Geometry: see drawing. Coordinates: mm, zero at the bounding-box minimum. A direction names the side the tool comes from. Give positions to 0.01 mm unless a question says otherwise; leave off trailing zeros. Order: outer loops, then holes, each group sorted by start corner. A loop starts at its lowest first (then second) coordinate and runs counter-clockwise, first axis right, second up. Notation, with made-up numbers: M -13.5,5.5 L 40.5,5.5 A32 cw 40.5,38.5 Z; hole C 42.5,18.5 d2. An arc over 180 degrees is marked long. Answer as a JSON object with one key per item and string values. Group by question number.
1. Section query D-D (x = 22.5). Output: boundary loops of the cut face in (y, z).
2. Pin query (flat end, axial travel): P1, Ø1.8, axis at x = 23, y = 22.25, coming from the +Z side; P2, Ø0.6, axis at x = 7.5, z = 0.5, coming from the -Y side; P3, Ø1, axis at y = 6.5, z = 1.5, coming from the -X side; P4, Ø0.6, axis at y = 12.5, z = 1, coming from the +X side. Return the tip coordinate at first contact, or that it passes through.
3. Section query A-A (x = 5). Output: boundary loops of the cut face in (y, z), plus the area to 3 significant figures.
4. Set-up query: the marked faces 1, 2 and 3. Return all of +Z, -Z, +X, -X, +Y, -Y with unobstructed straight access to the full face (end or side cutting, diameter ignored); none if empty.
5. Pull-direction query (Y, two-part tool) for the marked faces 4, 5 and 6; classes: +Y half, -Y half, draft (parallel to the pull), parting line (faces both ways), or undercut.
6. Section query C-C (z = 1.1). Output: boundary loops of the cut face in (x, y), plus the area to 3 significant figures.
7. Material intervals for L1, parallel to Y at x = 23, z = 0.95; L2, parallel to X at y = 23, z = 1.05; L3, parallel to X at y = 1.75, z = 0.65, sorted ascending. Write a range as [from, to].
8. Section query B-B (y = 22.25). Output: boundary loops of the cut face in (x, z).
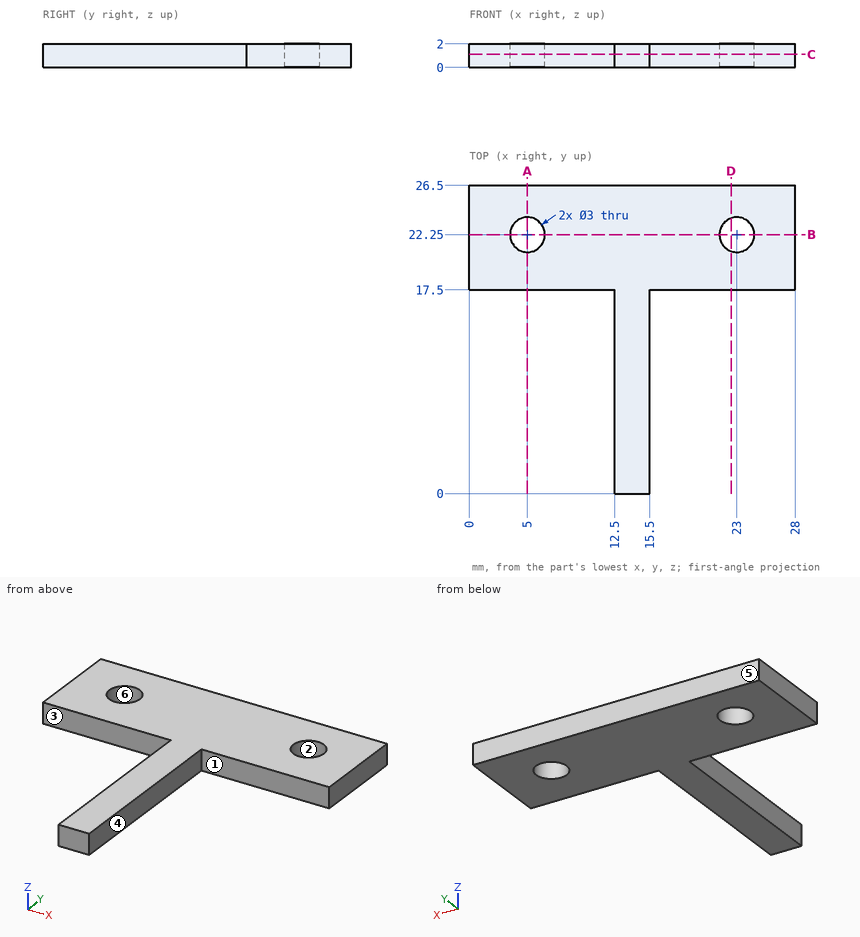
Answer sheet:
{
 "1": {"outline": "M 17.5,0 L 20.84,0 L 20.84,2 L 17.5,2 Z; M 23.66,0 L 26.5,0 L 26.5,2 L 23.66,2 Z"},
 "2": {"P1": "through", "P2": "y = 17.5", "P3": "x = 12.5", "P4": "x = 15.5"},
 "3": {"outline": "M 17.5,0 L 20.75,0 L 20.75,2 L 17.5,2 Z; M 23.75,0 L 26.5,0 L 26.5,2 L 23.75,2 Z", "area": "12.0 mm^2"},
 "4": {"face 1": "+Z, -Z, +X, -Y", "face 2": "+Z, -Z", "face 3": "+Z, -Z, -X, -Y"},
 "5": {"face 4": "draft", "face 5": "+Y half", "face 6": "undercut"},
 "6": {"outline": "M 0,17.5 L 12.5,17.5 L 12.5,0 L 15.5,0 L 15.5,17.5 L 28,17.5 L 28,26.5 L 0,26.5 Z; hole C 5,22.25 d3; hole C 23,22.25 d3", "area": "290 mm^2"},
 "7": {"L1": "[17.5, 20.75], [23.75, 26.5]", "L2": "[0, 3.7], [6.3, 21.7], [24.3, 28]", "L3": "[12.5, 15.5]"},
 "8": {"outline": "M 0,0 L 3.5,0 L 3.5,2 L 0,2 Z; M 6.5,0 L 21.5,0 L 21.5,2 L 6.5,2 Z; M 24.5,0 L 28,0 L 28,2 L 24.5,2 Z"}
}
